```python
from build123d import *

# Parameters (mm, degrees)
BOSS_EXTRUDE1_DEPTH = 70
CUT_EXTRUDE1_DEPTH  = 65
SKETCH5_R           = 8
CUT_EXTRUDE2_DEPTH  = 10
SKETCH6_R           = 8
CUT_EXTRUDE3_DEPTH  = 10
CHAMFER2_SIZE       = 1
SKETCH7_W           = 11
SKETCH7_H           = 11
CUT_EXTRUDE4_DEPTH  = 10
SKETCH8_W           = 11
SKETCH8_H           = 11
CUT_EXTRUDE5_DEPTH  = 10
SKETCH9_W           = 13
SKETCH9_H           = 10
BOSS_EXTRUDE2_DEPTH = 6
SKETCH10_R          = 2
CUT_EXTRUDE6_DEPTH  = 10
FILLET1_R           = 5


with BuildPart() as part:
    # Sketch1 → Boss-Extrude1 (new body)
    with BuildSketch(Plane(origin=(0, 0, 0), x_dir=(1, 0, 0), z_dir=(0, 1, 0))):
        Polygon((57.735026919, -100), (100, -57.735026919), (-100, -57.735026919), (-57.735026919, -100), (0, -115.470053838), align=None)
    extrude(amount=BOSS_EXTRUDE1_DEPTH)

    # Sketch4 → Cut-Extrude1 (cut)
    with BuildSketch(Plane(origin=(0, 70, 0), x_dir=(1, 0, 0), z_dir=(0, 1, 0))):
        Polygon((110.293672936, 0), (95.517122639, 55.146836468), (55.146836468, 95.517122639), (0, 110.293672936), (-55.146836468, 95.517122639), (-95.517122639, 55.146836468), (-110.293672936, 0), (-95.517122639, -55.146836468), (-55.146836468, -95.517122639), (0, -110.293672936), (55.146836468, -95.517122639), (95.517122639, -55.146836468), align=None)
    extrude(amount=-CUT_EXTRUDE1_DEPTH, mode=Mode.SUBTRACT)

    # Sketch5 → Cut-Extrude2 (cut)
    with BuildSketch(Plane(origin=(-28.867513459, 0, 107.735026919), x_dir=(0.9659258262890683, 0, 0.25881904510252085), z_dir=(-0.2588190451025208, 0, 0.9659258262890682))):
        with Locations((10.114150928, 43)):
            Circle(SKETCH5_R)
        with Locations((10.114150928, 17)):
            Circle(SKETCH5_R)
    extrude(amount=-CUT_EXTRUDE2_DEPTH, mode=Mode.SUBTRACT)

    # Sketch6 → Cut-Extrude3 (cut)
    with BuildSketch(Plane(origin=(28.867513459, 0, 107.735026919), x_dir=(0.9659258262890683, 0, -0.25881904510252085), z_dir=(0.2588190451025208, 0, 0.9659258262890682))):
        with Locations((-9.885849072, 17)):
            Circle(SKETCH6_R)
        with Locations((-9.885849072, 43)):
            Circle(SKETCH6_R)
    extrude(amount=-CUT_EXTRUDE3_DEPTH, mode=Mode.SUBTRACT)

    # Chamfer2
    chamfer2_edges = [part.edges().sort_by_distance(p)[0] for p in [
        (-26.825400478, 43, 108.282209443),
        (-26.825400478, 17, 108.282209443),
        (11.591109915, 17, 112.364225297),
        (11.591109915, 43, 112.364225297),
    ]]
    chamfer(chamfer2_edges, length=CHAMFER2_SIZE)

    # Sketch7 → Cut-Extrude4 (cut)
    with BuildSketch(Plane(origin=(-28.867513459, 0, 107.735026919), x_dir=(0.9659258262890683, 0, 0.25881904510252085), z_dir=(-0.2588190451025208, 0, 0.9659258262890682))):
        with Locations((-14.385849072, 28)):
            Rectangle(SKETCH7_W, SKETCH7_H)
    extrude(amount=-CUT_EXTRUDE4_DEPTH, mode=Mode.SUBTRACT)

    # Sketch8 → Cut-Extrude5 (cut)
    with BuildSketch(Plane(origin=(28.867513459, 0, 107.735026919), x_dir=(0.9659258262890683, 0, -0.25881904510252085), z_dir=(0.2588190451025208, 0, 0.9659258262890682))):
        with Locations((14.385849072, 28)):
            Rectangle(SKETCH8_W, SKETCH8_H)
    extrude(amount=-CUT_EXTRUDE5_DEPTH, mode=Mode.SUBTRACT)

    # Sketch9 → Boss-Extrude2 (add)
    with BuildSketch(Plane(origin=(0, 0, 57.735026919), x_dir=(-1, 0, 0), z_dir=(0, 0, -1))):
        with Locations((-26.5, 10)):
            Rectangle(SKETCH9_W, SKETCH9_H)
        with Locations((26.5, 10)):
            Rectangle(SKETCH9_W, SKETCH9_H)
    extrude(amount=-BOSS_EXTRUDE2_DEPTH)

    # Sketch10 → Cut-Extrude6 (cut)
    with BuildSketch(Plane(origin=(0, 0, 57.735026919), x_dir=(-1, 0, 0), z_dir=(0, 0, -1))):
        with Locations((-26.5, 11)):
            Circle(SKETCH10_R)
        with Locations((26.5, 11)):
            Circle(SKETCH10_R)
    extrude(amount=-CUT_EXTRUDE6_DEPTH, mode=Mode.SUBTRACT)

    # Fillet1
    fillet1_edges = [part.edges().sort_by_distance(p)[0] for p in [
        (-33, 5, 60.735026919),
        (-20, 5, 60.735026919),
        (20, 5, 60.735026919),
        (33, 5, 60.735026919),
    ]]
    fillet(fillet1_edges, radius=FILLET1_R)
    fillet1_2_edges = [part.edges().sort_by_distance(p)[0] for p in [
        (-33, 15, 60.735026919),
        (-20, 15, 60.735026919),
        (20, 15, 60.735026919),
        (33, 15, 60.735026919),
    ]]
    fillet(fillet1_2_edges, radius=FILLET1_R - 0.0001)  # a hair under: the kernel refuses the full size


solid = part.part
```
Check sheet for the modelled part. Datum: model origin and axes. Units: mm. A direction names the side the tool comes from. Round coordinates to 2 decimals unless told otherwise and drop trailing zeros. Order: outer loops, then holes, each group sorted by start corner. A loop starts at its lowest first (then second) coordinate and runs counter-clockwise, first axis right, second up.
1) Mould release check, pull along Z, two halves, no side actions. Record for faces 6 (the cylindrical face through (-28.408, 11.601, 60.693)), 7 (the flat face through (78.572, 34.51, 79.163)), 8 (the flat face through (73.773, 37.955, 76.891)), 9 (the flat face through (-26, 8, 63.735)): +Z half, -Z half, draft (parallel to the pull), parting line (faces both ways), or undercut.
2) Scan lines: line 1 (Y direction, x = -26.5, z = 61.75); line 2 (X direction, y = 21, z = 70); line 3 (X direction, y = 7, z = 89.5). Record each from-to range of solid material in increasing order.
3) Section check A-A (y = 65.5). Record the boundary of the cut face in (x, z).
4) Section check C-C (z = 71.5). Record the boundary of the cut face in (x, y).
5) Tool access check on faces 1 (the flat face through (47.44, 27.92, 100.21)), 2 (the flat face through (-29.272, 34.51, 107.627)), 3 (the flat face through (27, 8, 63.735)), 4 (the flat face through (-74.302, 37.955, 76.362)), 5 (the cylindrical face through (-11.191, 13.936, 109.395)). Record the directions out of +Z, -Z, +X, -X, +Y, -Y that give a thin tool (end or side, any length) a straight path to the whole face; none if there is none.
6) Go/stop test with flat-tipped pins: pin 1 Ø12 at (y, z) = (9.5, 75.5) entering from -X (3 decimals); pin 2 Ø4 at (x, z) = (31.5, 65.5) entering from +Y; pin 3 Ø3 at (x, y) = (-23.5, 8) entering from +Z. Record where each tip stops, or that it passes through.
7) Section check D-D (y = 19.5). Give the number of separate pieces and of enclosed holes in the cut face, and give its area (3 significant figures).
8) Section check B-B (x = -41). Record the boundary of the cut face in (y, z), and give its area (3 significant figures).
Result:
1. face 6: draft
1. face 7: +Z half
1. face 8: -Z half
1. face 9: undercut
2. line 1: y = 0 to 9, 13 to 15
2. line 2: x = -87.74 to -80.66, 80.66 to 87.74
2. line 3: x = -68.24 to -61.16, 61.16 to 68.24
3. outline: (-100, 57.74) - (-92.93, 57.74) - (-55.15, 95.52) - (0, 110.29) - (55.15, 95.52) - (92.93, 57.74) - (100, 57.74) - (57.74, 100) - (0, 115.47) - (-57.74, 100) - close
4. outline: (-86.24, 0) - (86.24, 0) - (86.24, 70) - (79.16, 70) - (79.16, 5) - (-79.16, 5) - (-79.16, 70) - (-86.24, 70) - close
5. face 1: +Z
5. face 2: +Z, -X, +Y, -Y
5. face 3: +Y
5. face 4: -Z, +Y
5. face 5: none
6. pin 1: stops at x = -88.235
6. pin 2: stops at y = 14.3
6. pin 3: stops at z = 109.58
7. separate pieces: 3
7. enclosed holes: 0
7. area: 996 mm2
8. outline: (0, 57.74) - (5, 57.74) - (5, 99.31) - (22.5, 99.31) - (22.5, 104.48) - (0, 104.48) - close; (33.5, 99.31) - (70, 99.31) - (70, 104.48) - (33.5, 104.48) - close
8. area: 513 mm2
